For this review, take the finished solid that the model builds, in its own axes (mm). A direction names the side the tool comes from. Coordinates: 2 decimals unless noted, no trailing zeros. Order: outer loops, then holes, each group sorted by start corner. A loop starts at its lowest first (then second) coordinate and runs counter-clockwise, first axis right, second up.
from build123d import *

# Parameters (mm, degrees)
SKETCH1_R           = 5
BOSS_EXTRUDE1_DEPTH = 13
CUT_EXTRUDE1_DEPTH  = 12
FILLET4_R           = 2
FILLET5_R           = 0.5
FILLET6_R           = 2


with BuildPart() as part:
    # Sketch1 → Boss-Extrude1 (new body)
    with BuildSketch(Plane(origin=(0, 0, 0), x_dir=(1, 0, 0), z_dir=(0, 1, 0))):
        with Locations(Location((0, 0, 0), (0, 0, 90))):
            Circle(SKETCH1_R)
    extrude(amount=BOSS_EXTRUDE1_DEPTH)

    # Insert → Cut-Extrude1 (cut)
    with BuildSketch(Plane.XZ):
        with BuildLine():
            Line((-1.75, 2.738612788), (-1.75, -2.738612788))
            ThreePointArc((-1.75, -2.738612788), (3.25, 0), (-1.75, 2.738612788))
        make_face()
    extrude(amount=-CUT_EXTRUDE1_DEPTH, mode=Mode.SUBTRACT)

    # Fillet4
    # the kernel refuses this fillet: 2 mm, written as the material it adds along each edge
    with BuildSketch(Plane(origin=(0, 12, 0), x_dir=(-0.9999950652018582, 0, -0.0031415874858799196), z_dir=(-0.0031415874858799196, 0, 0.9999950652018582))) as fillet4_piece_1:
        with BuildLine():
            CenterArc((3.25 - FILLET4_R, FILLET4_R), FILLET4_R, 270, 90)
            Line((3.25 - FILLET4_R, 0), (3.25, 0))
            Line((3.25, 0), (3.25, FILLET4_R))
        make_face()
    revolve(axis=Axis((0, 12, 0), (0, -1, 0)), revolution_arc=359.64)
    with BuildSketch(Plane(origin=(-1.75, 12, 7.738612788), x_dir=(0, -1, 0), z_dir=(0, 0, -1))) as fillet4_piece_2_section:
        with BuildLine():
            CenterArc((FILLET4_R, -FILLET4_R), FILLET4_R, 90, 90)
            Line((0, -FILLET4_R), (0, 0))
            Line((0, 0), (FILLET4_R, 0))
        make_face()
    fillet4_piece_2 = extrude(amount=15.477225575, mode=Mode.PRIVATE)
    fillet4_piece_2 = fillet4_piece_2 & Plane(origin=(0, 11.564510451, 0), x_dir=(-0.5384615384615385, 0, -0.8426500884694863), z_dir=(0, -1, 0)) * Cylinder(3.25, 39, mode=Mode.PRIVATE)
    add(fillet4_piece_2)

    # Fillet5
    fillet5_edges = [part.edges().sort_by_distance(p)[0] for p in [
        (3.25, 0, 0),
        (-1.75, 0, 0),
    ]]
    fillet(fillet5_edges, radius=FILLET5_R)

    # Fillet6
    fillet6_edges = [part.edges().sort_by_distance(p)[0] for p in [
        (0, 13, 5),
    ]]
    fillet(fillet6_edges, radius=FILLET6_R)


solid = part.part
1. Machinability: for faces 1 (the face through (-3, 0, 0)), 2 (the face through (-1.75, 5, 0)), which of the approach directions +Z, -Z, +X, -X, +Y, -Y give a long, thin tool a straight path to every point of the face, cutting with its end or side? Answer none if there is none.
Answer below:
face 1: +Z, -Z, +X, -X, -Y
face 2: -Y
2. To check wall thickness, follow L1, parallel to X at y = 8, z = 0; L2, parallel to Z at x = 1.75, y = 1; L3, parallel to Z at x = -4, y = 4.75. State the ranges of each line that lie inside material, in increasing order.
Answer below:
L1: x = -5 to -1.75, 3.25 to 5
L2: z = -4.68 to -2.74, 2.74 to 4.68
L3: z = -3 to 3
3. The part is to be moulded in two halves that separate along X. For faces 3 (the face through (3.25, 5.18, -0.1)), 4 (the face through (0, 13, 0)), 5 (the face through (4.88, 5.42, 1.08)), say which applies: +X half, -X half, draft (parallel to the pull), parting line (faces both ways), or undercut.
Answer below:
face 3: undercut
face 4: draft
face 5: parting line
4. Take a section at A-A, the plane y = 3.5. Give the boundary of the cut face in (x, z).
Answer below:
outline: circle Ø10 at (0, 0); hole (-1.75, -2.74) arc R3.25 ccw (long way) to (-1.75, 2.74) - close
5. Clearance check with flat-ended pins moving along their axes: pin 1 Ø1.5 at (x, y) = (3.5, 4) entering from -Z; pin 2 Ø5 at (x, y) = (3.5, 7.5) entering from -Z; pin 3 Ø3 at (y, z) = (8, -3) entering from -X. State where each tip first meets the part, or that it passes through.
Answer below:
pin 1: stops at z = -4.18
pin 2: stops at z = -4.9
pin 3: stops at x = -4.77
